The listing builds one solid part. Answer for the finished solid, in the listing's coordinates (mm). A direction names the side the tool comes from. Round coordinates to 2 decimals unless told otherwise and drop trailing zeros. Order: outer loops, then holes, each group sorted by start corner. A loop starts at its lowest first (then second) coordinate and runs counter-clockwise, first axis right, second up. Notation, with made-up numbers: (45.5, -13) -> (76.5, -13) arc R28 ccw to (76.5, 25) -> close; hole circle Ø10 at (-19.75, 17). An arc over 180 degrees is marked (long way). Answer in a Markdown table with one row per item. Add a question column.
```python
from build123d import *

# Parameters (mm, degrees)
EXTRUDE_1_DEPTH              = 3
SKETCH_2_W                   = 13.6
SKETCH_2_H                   = 29
CUT_EXTRUDE_1_DEPTH          = 1.7
SKETCH_3_W                   = 11.8
SKETCH_3_H                   = 22.7
CUT_EXTRUDE_2_DEPTH          = 4
HOLE_WIZARD_M3_1_D           = 3.4
HOLE_WIZARD_M3_1_DEPTH       = 7.5
HOLE_WIZARD_M3_1_CBORE_D     = 5.5
HOLE_WIZARD_M3_1_CBORE_DEPTH = 0.5
HOLE_WIZARD_M3_1_TIP         = 1.021463052
CHAMFER_1_SIZE               = 1
FILLET_1_R                   = 2
FILLET_3_R                   = 1


with BuildPart() as part:
    # 草图1 → 凸台-拉伸1 (new body)
    with BuildSketch(Plane.XY):
        Polygon((-7.7, -32), (25.3, -32), (25.3, -24), (17.6, -24), (17.6, 0), (0, 0), (0, -24), (-7.7, -24), align=None)
    extrude(amount=EXTRUDE_1_DEPTH)

    # 草图2 → 切除-拉伸1 (cut)
    with BuildSketch(Plane(origin=(0, 0, 0), x_dir=(-1, 0, 0), z_dir=(0, 0, -1))):
        with Locations((-8.8, -15.5)):
            Rectangle(SKETCH_2_W, SKETCH_2_H)
    extrude(amount=-CUT_EXTRUDE_1_DEPTH, mode=Mode.SUBTRACT)

    # 草图3 → 切除-拉伸2 (cut, through all)
    with BuildSketch(Plane.XY.offset(3)):
        with Locations((8.8, -13.55)):
            Rectangle(SKETCH_3_W, SKETCH_3_H)
    extrude(amount=-CUT_EXTRUDE_2_DEPTH, mode=Mode.SUBTRACT)

    # M3 六角头螺栓的柱形沉头孔1
    with Locations(Plane.XY.offset(3)):
        with Locations((-3.7, -28), (21.3, -28)):
            CounterBoreHole(HOLE_WIZARD_M3_1_D / 2, HOLE_WIZARD_M3_1_CBORE_D / 2, HOLE_WIZARD_M3_1_CBORE_DEPTH, depth=HOLE_WIZARD_M3_1_DEPTH)
            with Locations((0, 0, -(HOLE_WIZARD_M3_1_DEPTH + HOLE_WIZARD_M3_1_TIP / 2))):  # 118° drill point
                Cone(0, HOLE_WIZARD_M3_1_D / 2, HOLE_WIZARD_M3_1_TIP, mode=Mode.SUBTRACT)

    # 倒角1
    chamfer_1_edges = [part.edges().sort_by_distance(p)[0] for p in [
        (0, 0, 1.5),
        (17.6, 0, 1.5),
        (25.3, -24, 1.5),
        (25.3, -32, 1.5),
        (-7.7, -32, 1.5),
        (-7.7, -24, 1.5),
    ]]
    chamfer(chamfer_1_edges, length=CHAMFER_1_SIZE)

    # 圆角1
    fillet_1_edges = [part.edges().sort_by_distance(p)[0] for p in [
        (17.6, -24, 1.5),
        (0, -24, 1.5),
    ]]
    fillet(fillet_1_edges, radius=FILLET_1_R)

    # 圆角3
    fillet_3_edges = [part.edges().sort_by_distance(p)[0] for p in [
        (2.9, -13.55, 3),
        (8.8, -24.9, 3),
        (14.7, -13.55, 3),
        (8.8, -2.2, 3),
    ]]
    fillet(fillet_3_edges, radius=FILLET_3_R)


solid = part.part
```
Item 1: A tool of negligible diameter and unlimited length cuts with its end or side. For faces 1 (the face through (9, -30, 1)), 2 (the face through (9, 0, 1)), 3 (the face through (17.6, -12, 1)), 4 (the face through (2.599, -13.377, 2.715)), 5 (the face through (0, -11, 1)), from which of +Z, -Z, +X, -X, +Y, -Y can it reach the whole face along a straight path? Write none if from no direction.
Item 2: The part is cut by section A-A, the plane x = -3.7. Give the vertices of the cut face in (y, z).
Item 3: The part is cut by section B-B, the plane z = 1.2. Give the vertices of the cut face in (x, y), and give its area (3 significant figures).
Item 4: For a pull along Y with two mould halves and no side action, classify faces 6 (the face through (-4.058, -25.273, 2.754)), 7 (the face through (9, -32, 1)), 8 (the face through (18.2, -23.43, 1.52)), 9 (the face through (15.001, -13.377, 2.715)) as released by +Y, released by -Y, zero draft, split by the parting line, or undercut.
Item 5: The part is cut by section C-C, the plane y = -28. Give the vertices of the cut face in (x, z), and give its area (3 significant figures).
Item 6: Find the intervals of material crossed by probe 1 along Y at (x, z) = (3, 1.25); probe 2 along Y at (x, z) = (21.3, 0.9); probe 3 along X at (y, z) = (-20.5, 1.2), in increasing order. Write a range as [from, to].
Item 7: Flat-ended cylindrical pins translate along their axes: P1, Ø1, axis at y = -14, z = 1, coming from the +X side; P2, Ø0.9, axis at x = 22.5, z = 1, coming from the +Y side. Find the tip coordinate at first contact, or state that the pin passes through.
Item 8: The part is cut by section D-D, the plane y = -3.5. Give the vertices of the cut face in (x, z), and give its area (3 significant figures).
Resolved:
| question | item | result |
|---|---|---|
| 1 | face 1 | -Z |
| 1 | face 2 | +Z, -Z, +X, -X, +Y |
| 1 | face 3 | +Z, -Z, +X, +Y |
| 1 | face 4 | +Z |
| 1 | face 5 | +Z, -Z, -X, +Y |
| 2 | outline | (-32, 0) -> (-29.7, 0) -> (-29.7, 2.5) -> (-30.75, 2.5) -> (-30.75, 3) -> (-32, 3) -> close; (-26.3, 0) -> (-24, 0) -> (-24, 3) -> (-25.25, 3) -> (-25.25, 2.5) -> (-26.3, 2.5) -> close |
| 3 | outline | (-7.7, -31) -> (-6.7, -32) -> (24.3, -32) -> (25.3, -31) -> (25.3, -25) -> (24.3, -24) -> (19.6, -24) arc R2 cw to (17.6, -22) -> (17.6, -1) -> (16.6, 0) -> (1, 0) -> (0, -1) -> (0, -22) arc R2 cw to (-2, -24) -> (-6.7, -24) -> (-7.7, -25) -> close; hole circle Ø3.4 at (-3.7, -28); hole (2, -30) -> (15.6, -30) -> (15.6, -1) -> (2, -1) -> close; hole circle Ø3.4 at (21.3, -28) |
| 3 | area | 273 mm2 |
| 4 | face 6 | undercut |
| 4 | face 7 | released by -Y |
| 4 | face 8 | released by +Y |
| 4 | face 9 | undercut |
| 5 | outline | (-7.7, 0) -> (-5.4, 0) -> (-5.4, 2.5) -> (-6.45, 2.5) -> (-6.45, 3) -> (-7.7, 3) -> close; (-2, 0) -> (2, 0) -> (2, 1.7) -> (15.6, 1.7) -> (15.6, 0) -> (19.6, 0) -> (19.6, 2.5) -> (18.55, 2.5) -> (18.55, 3) -> (-0.95, 3) -> (-0.95, 2.5) -> (-2, 2.5) -> close; (23, 0) -> (25.3, 0) -> (25.3, 3) -> (24.05, 3) -> (24.05, 2.5) -> (23, 2.5) -> close |
| 5 | area | 53.4 mm2 |
| 6 | probe 1 | [-32, -30], [-1, 0] |
| 6 | probe 2 | [-32, -29.7], [-26.3, -24] |
| 6 | probe 3 | [0, 2], [15.6, 17.6] |
| 7 | P1 | x = 17.6 |
| 7 | P2 | y = -24 |
| 8 | outline | (0, 0) -> (2, 0) -> (2, 1.7) -> (2.9, 1.7) -> (2.9, 2) arc R1 ccw to (1.9, 3) -> (0, 3) -> close; (14.7, 1.7) -> (15.6, 1.7) -> (15.6, 0) -> (17.6, 0) -> (17.6, 3) -> (15.7, 3) arc R1 ccw to (14.7, 2) -> close |
| 8 | area | 13.9 mm2 |
